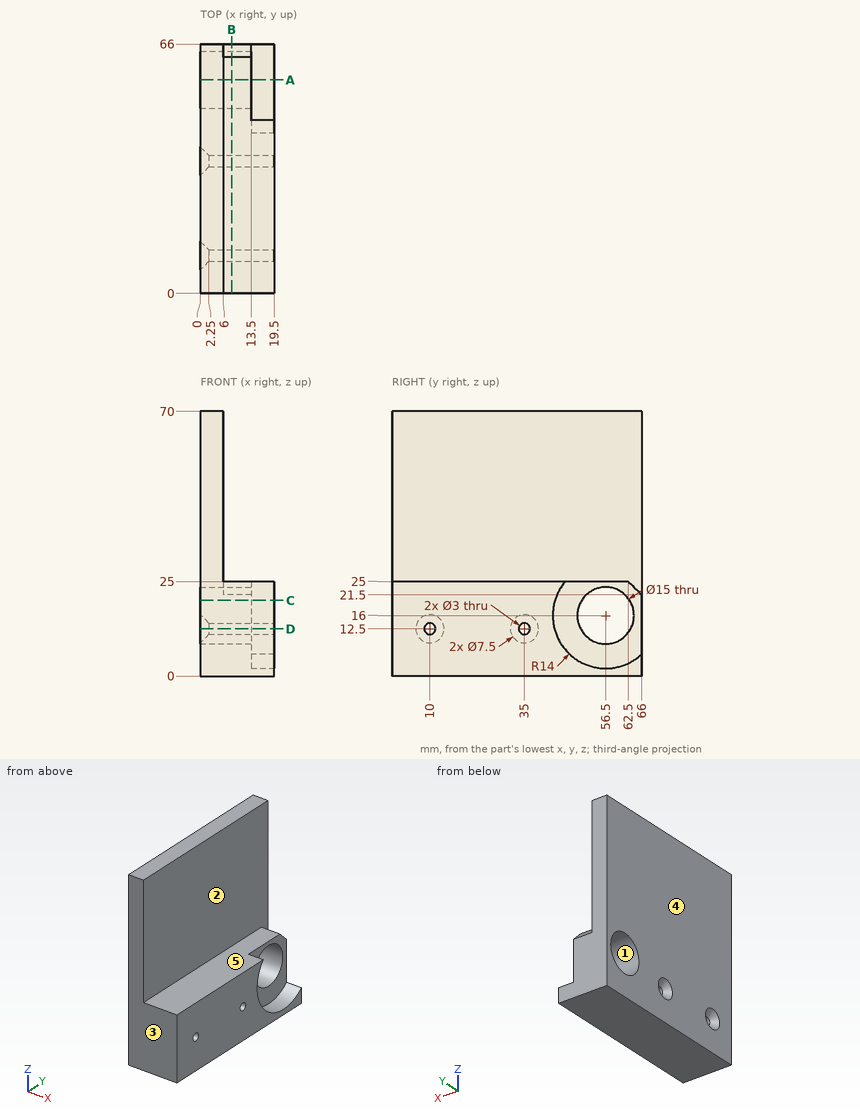
Can you work these out from the drawing? Everything is in mm from the part's minimum corner. A direction names the side the tool comes from. Give positions to 0.01 mm unless a question says otherwise; leave off trailing zeros. Loops run counter-clockwise (first coordinate to the right, second up) from the corner with the lowest first, then second, coordinate; pieces in that order, holes last. Notation, with made-up numbers: (2, 31.25) -> (26, 31.25) arc R27 cw to (26, 61.25) -> close; hole circle Ø4 at (18.25, 82.5). An arc over 180 degrees is marked (long way). Put each result on its own line as item: value.
(1) Thinking about a two-plate mould opening in Y: for the marked faces 1, 2 and 3, which applies, pulls with the +Y half, pulls with the -Y half, needs draft (parallel to the pull), parting line crosses it, or undercut?
Computed:
face 1: undercut
face 2: needs draft
face 3: pulls with the -Y half
(2) Imagine slicing it at D-D on z = 12.5. Write out the boundary of the cut face in (x, y).
Computed:
outline: (0, 0) -> (19.5, 0) -> (19.5, 8.5) -> (2.25, 8.5) -> (0, 6.25) -> close; (0, 13.75) -> (2.25, 11.5) -> (19.5, 11.5) -> (19.5, 33.5) -> (2.25, 33.5) -> (0, 31.25) -> close; (0, 38.75) -> (2.25, 36.5) -> (19.5, 36.5) -> (19.5, 42.94) -> (13.5, 42.94) -> (13.5, 49.87) -> (0, 49.87) -> close; (0, 63.13) -> (13.5, 63.13) -> (13.5, 66) -> (0, 66) -> close
(3) Imagine slicing it at A-A on y = 56.5. Write out the boundary of the cut face in (x, z), plus the area to 3 significant figures.
Computed:
outline: (0, 0) -> (19.5, 0) -> (19.5, 2) -> (13.5, 2) -> (13.5, 8.5) -> (0, 8.5) -> close; (0, 23.5) -> (13.5, 23.5) -> (13.5, 25) -> (6, 25) -> (6, 70) -> (0, 70) -> close
area: 417 mm^2
(4) Imagine slicing it at B-B on x = 8.25. Write out the boundary of the cut face in (y, z).
Computed:
outline: (0, 0) -> (66, 0) -> (66, 21.5) -> (62.5, 25) -> (0, 25) -> close; hole circle Ø3 at (10, 12.5); hole circle Ø3 at (35, 12.5); hole circle Ø15 at (56.5, 16)
(5) Imagine slicing it at C-C on z = 20. Write out the boundary of the cut face in (x, y), plus the area to 3 significant figures.
Computed:
outline: (0, 0) -> (19.5, 0) -> (19.5, 43.08) -> (13.5, 43.08) -> (13.5, 50.16) -> (0, 50.16) -> close; (0, 62.84) -> (13.5, 62.84) -> (13.5, 66) -> (0, 66) -> close
area: 978 mm^2
(6) Please list where these lines run through material, in increasing order: probe 1 along Z at (x, y) = (10.5, 57); probe 2 along Z at (x, y) = (14.5, 10); probe 3 along Y at (x, z) = (9.75, 12.5). Write a range as [from, to].
Computed:
probe 1: [0, 8.52], [23.48, 25]
probe 2: [0, 11], [14, 25]
probe 3: [0, 8.5], [11.5, 33.5], [36.5, 49.87], [63.13, 66]
(7) For the marked faces 4 and 5, which set-ups out of +Z, -Z, +X, -X, +Y, -Y let a thin tool reach every point of the face, with its end or its side?
Computed:
face 4: +Z, -Z, -X, +Y, -Y
face 5: +Z, +X, +Y, -Y
(8) I'm going to push flat-ended pins straight in: pin 1 Ø14.5 at (y, z) = (17, 40.5) entering from +X; pin 2 Ø3 at (x, y) = (11, 22.5) entering from +Z; pin 3 Ø11 at (x, y) = (10.5, 46.5) entering from +Z. Where does each tip first touch, or does it pass through?
Computed:
pin 1: x = 6
pin 2: z = 25
pin 3: z = 70
